Autodesk Inventor part; units mm, degrees
ref_plane "YZ Plane" through (0, 0, 0) normal (1, 0, 0) x (0, 1, 0)
ref_plane "XZ Plane" through (0, 0, 0) normal (0, 1, 0) x (-1, 0, 0)
ref_plane "XY Plane" through (0, 0, 0) normal (0, 0, 1) x (1, 0, 0)
sketch "Sketch1" plane through (0, 0, 0) normal (0, 0, 1) x (1, 0, 0)
  line L0 (-63.5, -22.225) -> (63.5, -22.225)
  line L1 (63.5, -22.225) -> (63.5, 22.225)
  line L2 (63.5, 22.225) -> (-63.5, 22.225)
  line L3 (-63.5, 22.225) -> (-63.5, -22.225)
  line L4 (-63.5, -22.225) -> (63.5, 22.225) construction
  line L5 (63.5, -22.225) -> (-63.5, 22.225) construction
  point P0 (0, 0)
  dimension "d0" = 127
  dimension "d1" = 44.45
extrude "Extrusion1" add sketch "Sketch1" along normal blind 4.7498
sketch "Sketch2" plane through (0, 0, 4.7498) normal (0, 0, 1) x (1, 0, 0)
  point P0 (0, 0)
sketch "Sketch3" plane through (0, 0, 4.7498) normal (0, 0, 1) x (1, 0, 0)
  line L0 (-63.5, -22.225) -> (63.5, -22.225) construction
  line L1 (63.5, -22.225) -> (63.5, 22.225) construction
  line L2 (63.5, 22.225) -> (-63.5, 22.225) construction
  line L3 (-63.5, 22.225) -> (-63.5, -22.225) construction
  line L4 (0, 22.225) -> (0, -22.225) construction
  circle A0 centre (-31.75, 0) radius 1.1303
  circle A1 centre (31.75, 0) radius 1.1303
  line L5 (-31.75, 0) -> (31.75, 0) construction
  line L6 (-26.0604, 5.334) -> (26.0604, 5.334)
  line L7 (-25.1841, -5.461) -> (25.1841, -5.461)
  arc A2 (29.3388, 1.2787) -> (26.0604, 5.334) centre (26.0604, 1.9812) ccw
  arc A3 (25.1841, -5.461) -> (28.4625, -2.8107) centre (25.1841, -2.1082) ccw
  arc A4 (-26.0604, 5.334) -> (-29.3388, 1.2787) centre (-26.0604, 1.9812) ccw
  line L8 (-29.3388, 1.2787) -> (-28.4625, -2.8107)
  line L9 (29.3388, 1.2787) -> (28.4625, -2.8107)
  arc A5 (-28.4625, -2.8107) -> (-25.1841, -5.461) centre (-25.1841, -2.1082) ccw
  line L10 (29.3388, 1.2787) -> (29.3388, -4.741) construction
  point P0 (0, 0)
  point P1 (0, 5.334)
  point P2 (0, -5.461)
  point P3 (-29.0648, 0)
  point P4 (-30.6197, 0)
  point P5 (-29.0648, 0)
  point P6 (-30.6197, 0)
  point P7 (-30.6197, 0)
  point P8 (-29.0648, 0)
  point P9 (29.0648, 0)
  dimension "d7" = 2.2606
  dimension "d8" = 2.2606
  dimension "d9" = 63.5
  dimension "d11" = 6.7056
  dimension "d13" = 6.7056
  dimension "d15" = 52.1208
  dimension "d16" = 50.3682
  dimension "d17" = 10.795
  dimension "d20" = 5.334
  dimension "d24" = 3.3528
  dimension "d25" = 3.3528
extrude "Extrusion2" cut sketch "Sketch3" against normal blind 4.7498
properties part number "dsub37_cutout"
For this review, take the finished solid that the model builds, in its own axes (mm). A direction names the side the tool comes from. Round coordinates to 2 decimals unless told otherwise and drop trailing zeros. Order: outer loops, then holes, each group sorted by start corner. A loop starts at its lowest first (then second) coordinate and runs counter-clockwise, first axis right, second up.
Q1. We need section A-A, the plane x = 13. Give the boundary of the cut face in (y, z) (3 decimals), plus the area to 3 significant figures.
Findings below:
outline: (-22.225, 0) - (-5.461, 0) - (-5.461, 4.75) - (-22.225, 4.75) - close; (5.334, 0) - (22.225, 0) - (22.225, 4.75) - (5.334, 4.75) - close
area: 160 mm2
Q2. Wall thickness on line 1 (Y direction, x = -31.75, z = 1.85) (3 decimals); line 2 (Y direction, x = 24, z = 2.7) (3 decimals); line 3 (X direction, y = -2, z = 3.6): over which ranges is each line inside the solid? List them lowest first.
Findings below:
line 1: y = -22.225 to -1.13, 1.13 to 22.225
line 2: y = -22.225 to -5.461, 5.334 to 22.225
line 3: x = -63.5 to -28.64, 28.64 to 63.5
Q3. We need section B-B, the plane z = 3.2. State how many separate pieces and enclosed holes the cut face has, plus the area to 3 significant figures.
Findings below:
separate pieces: 1
enclosed holes: 3
area: 5,020 mm2
Q4. Machinability: for faces 5 (the flat face through (1, 22.225, 2)), 6 (the cylindrical face through (-27.317, -4.695, 2.408)), which of the approach directions +Z, -Z, +X, -X, +Y, -Y give a long, thin tool a straight path to every point of the face, cutting with its end or side? Answer none if there is none.
Findings below:
face 5: +Z, -Z, +X, -X, +Y
face 6: +Z, -Z
Q5. Mouldability with a two-part tool opening along Y and no side actions: class faces 1 (the flat face through (-1, -22.225, 2)), 2 (the cylindrical face through (28.69, 4.06, 2.41)), 3 (the flat face through (-63.5, 0, 2)), 4 (the flat face through (28.907, -0.737, 2.408)) as pulls with the +Y half, pulls with the -Y half, needs draft (parallel to the pull), parting line crosses it, or undercut.
Findings below:
face 1: pulls with the -Y half
face 2: undercut
face 3: needs draft
face 4: undercut
Q6. We need section D-D, the plane x = 31.75. Give the boundary of the cut face in (y, z) (3 decimals), plus the area to 3 significant figures.
Findings below:
outline: (-22.225, 0) - (-1.13, 0) - (-1.13, 4.75) - (-22.225, 4.75) - close; (1.13, 0) - (22.225, 0) - (22.225, 4.75) - (1.13, 4.75) - close
area: 200 mm2
Q7. We need section C-C, the plane y = 0. Give the boundary of the cut face in (x, z), plus the area to 3 significant figures.
Findings below:
outline: (-63.5, 0) - (-32.88, 0) - (-32.88, 4.75) - (-63.5, 4.75) - close; (-30.62, 0) - (-29.06, 0) - (-29.06, 4.75) - (-30.62, 4.75) - close; (29.06, 0) - (30.62, 0) - (30.62, 4.75) - (29.06, 4.75) - close; (32.88, 0) - (63.5, 0) - (63.5, 4.75) - (32.88, 4.75) - close
area: 306 mm2
